from build123d import *

# Parameters (mm, degrees)
SKETCH1_R           = 31.0896
BOSS_EXTRUDE1_DEPTH = 16.002
BOSS_EXTRUDE2_START = -6.35
BOSS_EXTRUDE2_DEPTH = 6.35
FILLET2_R           = 6.35
CUT_EXTRUDE2_REACH  = 96.198
SKETCH4_R           = 1.778
SKETCH4_R_2         = 6.35
SKETCH7_R           = 2.0193
CUT_EXTRUDE4_DEPTH  = 95.197625109
FILLET7_R           = 6.35
FILLET8_R           = 41.148
CUT_EXTRUDE5_DEPTH  = 12.7
FILLET9_R           = 2.54
SKETCH9_R           = 6.35
CUT_EXTRUDE6_DEPTH  = 3.302
FILLET10_R          = 3.556


# Some blends are built 0.0001 mm under size
with BuildPart() as part:
    # Sketch1 → Boss-Extrude1 (new body)
    with BuildSketch(Plane(origin=(0, 0, 0), x_dir=(1, 0, 0), z_dir=(0, 1, 0))):
        with Locations(Location((0, 0, 0), (0, 0, 270))):
            Circle(SKETCH1_R)
    extrude(amount=BOSS_EXTRUDE1_DEPTH)

    # Sketch2 → Boss-Extrude2 (add)
    with BuildSketch(Plane(origin=(0, 16.002, 0), x_dir=(1, 0, 0), z_dir=(0, 1, 0)).offset(BOSS_EXTRUDE2_START)):
        with BuildLine():
            Line((-31.0896, 0), (-31.0896, 41.148))
            Line((-31.0896, 41.148), (83.2104, 41.148))
            Line((83.2104, 41.148), (83.2104, 15.748))
            Line((83.2104, 15.748), (31.0896, 15.748))
            Line((31.0896, 15.748), (31.0896, 0))
            ThreePointArc((31.0896, 0), (0, -31.0896), (-31.0896, 0))
        make_face()
    extrude(amount=BOSS_EXTRUDE2_DEPTH)

    # Fillet2
    fillet2_edges = [part.edges().sort_by_distance(p)[0] for p in [
        (31.0896, 12.827, -15.748),
    ]]
    fillet(fillet2_edges, radius=FILLET2_R)

    # Sketch4 → Cut-Extrude2 (cut, up to next)
    with BuildSketch(Plane(origin=(0, 16.002, 0), x_dir=(1, 0, 0), z_dir=(0, 1, 0)), mode=Mode.PRIVATE) as cut_extrude2_sk1:
        with Locations(Location((61.411202787, 35.362797213, 0), (0, 0, 270))):
            Circle(SKETCH4_R)
    cut_extrude2_tool1 = extrude(cut_extrude2_sk1.sketch, amount=-CUT_EXTRUDE2_REACH, mode=Mode.PRIVATE) & part.part
    # Sketch4 → Cut-Extrude2 (cut, up to next)
    with BuildSketch(Plane(origin=(0, 16.002, 0), x_dir=(1, 0, 0), z_dir=(0, 1, 0)), mode=Mode.PRIVATE) as cut_extrude2_sk2:
        with Locations(Location((75.240797213, 35.362797213, 0), (0, 0, 270))):
            Circle(SKETCH4_R)
    cut_extrude2_tool2 = extrude(cut_extrude2_sk2.sketch, amount=-CUT_EXTRUDE2_REACH, mode=Mode.PRIVATE) & part.part
    # Sketch4 → Cut-Extrude2 (cut, up to next)
    with BuildSketch(Plane(origin=(0, 16.002, 0), x_dir=(1, 0, 0), z_dir=(0, 1, 0)), mode=Mode.PRIVATE) as cut_extrude2_sk3:
        with Locations(Location((75.240797213, 21.533202787, 0), (0, 0, 270))):
            Circle(SKETCH4_R)
    cut_extrude2_tool3 = extrude(cut_extrude2_sk3.sketch, amount=-CUT_EXTRUDE2_REACH, mode=Mode.PRIVATE) & part.part
    # Sketch4 → Cut-Extrude2 (cut, up to next)
    with BuildSketch(Plane(origin=(0, 16.002, 0), x_dir=(1, 0, 0), z_dir=(0, 1, 0)), mode=Mode.PRIVATE) as cut_extrude2_sk4:
        with Locations(Location((68.326, 28.448, 0), (0, 0, 270))):
            Circle(SKETCH4_R_2)
    cut_extrude2_tool4 = extrude(cut_extrude2_sk4.sketch, amount=-CUT_EXTRUDE2_REACH, mode=Mode.PRIVATE) & part.part
    # Sketch4 → Cut-Extrude2 (cut, up to next)
    with BuildSketch(Plane(origin=(0, 16.002, 0), x_dir=(1, 0, 0), z_dir=(0, 1, 0)), mode=Mode.PRIVATE) as cut_extrude2_sk5:
        with Locations(Location((61.411202787, 21.533202787, 0), (0, 0, 270))):
            Circle(SKETCH4_R)
    cut_extrude2_tool5 = extrude(cut_extrude2_sk5.sketch, amount=-CUT_EXTRUDE2_REACH, mode=Mode.PRIVATE) & part.part
    add(cut_extrude2_tool1.solids().sort_by_distance((61.411203, 16.002, -35.362797))[0], mode=Mode.SUBTRACT)
    add(cut_extrude2_tool2.solids().sort_by_distance((75.240797, 16.002, -35.362797))[0], mode=Mode.SUBTRACT)
    add(cut_extrude2_tool3.solids().sort_by_distance((75.240797, 16.002, -21.533203))[0], mode=Mode.SUBTRACT)
    add(cut_extrude2_tool4.solids().sort_by_distance((68.326, 16.002, -28.448))[0], mode=Mode.SUBTRACT)
    add(cut_extrude2_tool5.solids().sort_by_distance((61.411203, 16.002, -21.533203))[0], mode=Mode.SUBTRACT)

    # Sketch7 → Cut-Extrude4 (cut, through all)
    with BuildSketch(Plane(origin=(0, 0, 0), x_dir=(1, 0, 0), z_dir=(0, 1, 0))):
        with BuildLine():
            ThreePointArc((27.94, 0), (22.235278576, 16.918510179), (7.450666667, 26.928259621))
            Line((7.450666667, 26.928259621), (4.402666667, 15.912153412))
            ThreePointArc((4.402666667, 15.912153412), (13.139028249, 9.997301469), (16.51, 0))
            ThreePointArc((16.51, 0), (13.139028249, -9.997301469), (4.402666667, -15.912153412))
            Line((4.402666667, -15.912153412), (7.450666667, -26.928259621))
            ThreePointArc((7.450666667, -26.928259621), (22.235278576, -16.918510179), (27.94, 0))
        make_face()
        with BuildLine():
            Line((-15.912153412, -4.402666667), (-26.928259621, -7.450666667))
            ThreePointArc((-26.928259621, -7.450666667), (-19.756563466, -19.756563466), (-7.450666667, -26.928259621))
            Line((-7.450666667, -26.928259621), (-4.402666667, -15.912153412))
            ThreePointArc((-4.402666667, -15.912153412), (-11.674332957, -11.674332957), (-15.912153412, -4.402666667))
        make_face()
        with BuildLine():
            Line((-4.402666667, 15.912153412), (-7.450666667, 26.928259621))
            ThreePointArc((-7.450666667, 26.928259621), (-19.756563466, 19.756563466), (-26.928259621, 7.450666667))
            Line((-26.928259621, 7.450666667), (-15.912153412, 4.402666667))
            ThreePointArc((-15.912153412, 4.402666667), (-11.674332957, 11.674332957), (-4.402666667, 15.912153412))
        make_face()
        with Locations(Location((-19.05, 0, 0), (0, 0, 270))):
            Circle(SKETCH7_R)
        with Locations(Location((0, -19.05, 0), (0, 0, 270))):
            Circle(SKETCH7_R)
        with Locations(Location((0, 19.05, 0), (0, 0, 270))):
            Circle(SKETCH7_R)
    extrude(amount=CUT_EXTRUDE4_DEPTH, mode=Mode.SUBTRACT)

    # Fillet7
    # the kernel refuses this fillet: 6.35 mm, written as the material it adds along each edge
    with BuildSketch(Plane(origin=(-26.928259621, 0, -7.450666667), x_dir=(0.40702884348062, 0, -0.9134153056385845), z_dir=(0, 1, 0)), Plane(origin=(-7.450666667, 0, 26.928259621), x_dir=(-0.9134153056385848, 0, -0.40702884348061963), z_dir=(0, 1, 0))) as fillet7_piece_1:
        with BuildLine():
            CenterArc((7.365726845, -6.279391075), FILLET7_R, 81.447682412, 107.104635177)
            Line((1.086335771, -7.223715029), (0, 0))
            ThreePointArc((0, 0), (4.1550254, 0.310679271), (8.3100508, 0))
        make_face()
    extrude(amount=16.002)
    with BuildSketch(Plane(origin=(-7.450666667, 0, -26.928259621), x_dir=(0.26666666666666705, 0, 0.9637888196533972), z_dir=(0, 1, 0)), Plane(origin=(7.450666667, 0, 26.928259621), x_dir=(-0.26666666666666733, 0, -0.9637888196533971), z_dir=(0, 1, 0)), Plane(origin=(-26.928259621, 0, 7.450666667), x_dir=(0.9637888196533975, 0, -0.26666666666666644), z_dir=(0, 1, 0))) as fillet7_piece_2:
        with BuildLine():
            CenterArc((7.304942452, -6.35), FILLET7_R, 90, 107.104635177)
            ThreePointArc((1.235807879, -8.217647059), (0.310679271, -4.1550254), (0, 0))
            Line((0, 0), (7.304942452, 0))
        make_face()
    extrude(amount=16.002)
    with BuildSketch(Plane(origin=(-4.402666667, 0, -15.912153412), x_dir=(-0.916852417954672, 0, 0.39922630636103035), z_dir=(0, 1, 0)), Plane(origin=(4.402666667, 0, 15.912153412), x_dir=(0.9168524179546733, 0, -0.39922630636102746), z_dir=(0, 1, 0)), Plane(origin=(-15.912153412, 0, 4.402666667), x_dir=(0.39922630636102946, 0, 0.9168524179546725), z_dir=(0, 1, 0))) as fillet7_piece_3:
        with BuildLine():
            CenterArc((5.522661099, -6.287214109), FILLET7_R, 98.063810107, 73.872379787)
            Line((-0.76455301, -5.396462319), (0, 0))
            ThreePointArc((0, 0), (2.315954654, -0.163243317), (4.631909309, 0))
        make_face()
    extrude(amount=16.002)
    with BuildSketch(Plane(origin=(4.402666667, 0, -15.912153412), x_dir=(0.26666666666666416, 0, -0.9637888196533979), z_dir=(0, 1, 0))) as fillet7_piece_4:
        with BuildLine():
            CenterArc((5.450352912, -6.35), FILLET7_R, 90, 73.872379787)
            ThreePointArc((-0.649745119, -4.586111111), (-0.163243317, -2.315954654), (0, 0))
            Line((0, 0), (5.450352912, 0))
        make_face()
    extrude(amount=16.002)
    with BuildSketch(Plane(origin=(7.450666667, 0, -26.928259621), x_dir=(-0.2666666666666666, 0, 0.9637888196533974), z_dir=(0, 1, 0))) as fillet7_piece_5:
        with BuildLine():
            CenterArc((7.304942452, 6.35), FILLET7_R, 162.895364823, 107.104635177)
            ThreePointArc((1.235807879, 8.217647059), (0.310679271, 4.1550254), (0, 0))
            Line((0, 0), (7.304942452, 0))
        make_face()
    extrude(amount=16.002)
    with BuildSketch(Plane(origin=(-4.402666667, 0, 15.912153412), x_dir=(-0.9168524179546729, 0, -0.3992263063610288), z_dir=(0, 1, 0)), Plane(origin=(-15.912153412, 0, -4.402666667), x_dir=(0.39922630636102996, 0, -0.9168524179546723), z_dir=(0, 1, 0))) as fillet7_piece_6:
        with BuildLine():
            CenterArc((5.522661099, 6.287214109), FILLET7_R, 188.063810107, 73.872379787)
            Line((-0.76455301, 5.396462319), (0, 0))
            ThreePointArc((0, 0), (2.315954654, 0.163243317), (4.631909309, 0))
        make_face()
    extrude(amount=16.002)

    # Fillet8
    fillet8_edges = [part.edges().sort_by_distance(p)[0] for p in [
        (-31.0896, 12.827, -41.148),
    ]]
    fillet(fillet8_edges, radius=FILLET8_R - 0.0001)  # a hair under: the kernel refuses the full size

    # Sketch8 → Cut-Extrude5 (cut)
    with BuildSketch(Plane.XZ):
        with BuildLine():
            Line((-10.414, 10.414), (10.414, 10.414))
            ThreePointArc((10.414, 10.414), (20.828, 0), (10.414, -10.414))
            Line((10.414, -10.414), (-10.414, -10.414))
            Line((-10.414, -10.414), (-10.414, 10.414))
        make_face()
    extrude(amount=-CUT_EXTRUDE5_DEPTH, mode=Mode.SUBTRACT)

    # Fillet9
    # the kernel refuses this fillet: 2.54 mm, written as the material it takes off along each edge
    with BuildSketch(Plane(origin=(13.087195122, 12.7, 10.065059555), x_dir=(-0.7525451578932851, 0, 0.658540648199768), z_dir=(0, -1, 0))) as fillet9_piece_1:
        with BuildLine():
            CenterArc((7.288242174, 2.538935053), FILLET9_R, 131.188669075, 137.152126286)
            Line((5.615548928, 4.450399754), (5.448279603, 4.641546224))
            ThreePointArc((5.448279603, 4.641546224), (2.074222188, 1.688960676), (-0.1125988, 0.227678524))
            Line((-0.1125988, 0.227678524), (-0.049545453, -0.249120951))
            ThreePointArc((-0.049545453, -0.249120951), (6.014734512, -0.336617786), (7.207343199, -0.253893505))
            Line((7.207343199, -0.253893505), (7.214697651, 0))
        make_face()
    extrude(amount=30.736744128, mode=Mode.SUBTRACT)
    with BuildSketch(Plane(origin=(13.087195122, 12.7, -10.065059555), x_dir=(-0.7525451578933744, 0, -0.658540648199666), z_dir=(0, -1, 0))) as fillet9_piece_2:
        with BuildLine():
            CenterArc((7.288242174, -2.538935053), FILLET9_R, 91.659204639, 137.152126286)
            Line((5.615548928, -4.450399754), (5.448279603, -4.641546224))
            ThreePointArc((5.448279603, -4.641546224), (2.074222188, -1.688960676), (-0.1125988, -0.227678524))
            Line((-0.1125988, -0.227678524), (-0.049545453, 0.249120951))
            ThreePointArc((-0.049545453, 0.249120951), (6.014734512, 0.336617786), (7.207343199, 0.253893505))
            Line((7.207343199, 0.253893505), (7.214697651, 0))
        make_face()
    extrude(amount=30.736744128, mode=Mode.SUBTRACT)

    # Sketch9 → Cut-Extrude6 (cut)
    with BuildSketch(Plane.XZ.offset(-12.7)):
        with Locations(Location((0, 0, 0), (0, 0, 270))):
            Circle(SKETCH9_R)
    extrude(amount=-CUT_EXTRUDE6_DEPTH, mode=Mode.SUBTRACT)

    # Fillet10
    fillet10_edges = [part.edges().sort_by_distance(p)[0] for p in [
        (-10.414, 6.35, -10.414),
        (-10.414, 6.35, 10.414),
    ]]
    fillet(fillet10_edges, radius=FILLET10_R)


solid = part.part
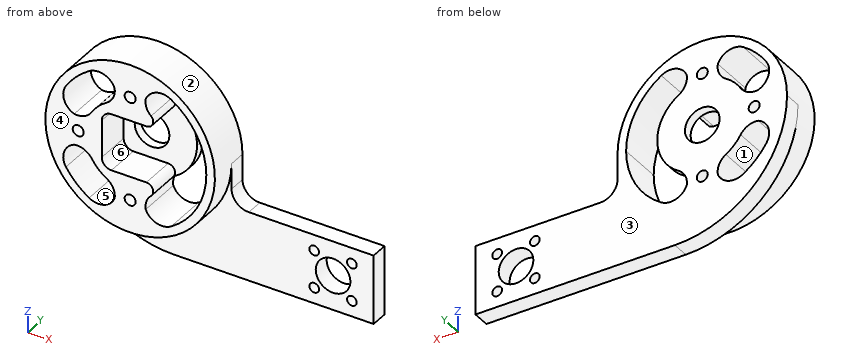
The listing builds one solid part. Answer for the finished solid, in the listing's coordinates (mm). Face numbers are marked on the shaded views. A direction names the side the tool comes from. Coordinates: 2 decimals unless noted, no trailing zeros. Loops run counter-clockwise (first coordinate to the right, second up) from the corner with the lowest first, then second, coordinate; pieces in that order, holes last. Notation, with made-up numbers: (85.25, 38.25) -> (123.25, 38.25) arc R30 ccw to (123.25, 69.25) -> close; hole circle Ø8 at (52, 31.25). An arc over 180 degrees is marked (long way). Write item = value, one per line. Start each with the question number.
1) A cutting plane is placed at C-C (x = -19.05). Give the vertices of the cut face in (y, z), then the cut area to 3 significant figures.
2) A cutting plane is placed at B-B (x = 12). Give the vertices of the cut face in (y, z).
3) The mould has two halves that part along X. Classify the marked faces 1, 2 and 3: released by +X, released by -X, zero draft, split by the parting line, or undercut.
4) Given pin 1 Ø4 at (y, z) = (7, -19.5) entering from +X; pin 2 Ø1.5 at (y, z) = (9.5, -3) entering from +X; pin 3 Ø5.5 at (x, z) = (75.24, -21.53) entering from +Y; pin 4 Ø4 at (x, z) = (61.41, -35.36) entering from -Y, each flat-ended and moving along its own axis, determine where each tip first touches the part or whether it passes through.
5) A cutting plane is placed at A-A (z = 19.05). Give the vertices of the cut face in (x, y), then the cut area to 3 significant figures.
6) Straight lines are drawn through the part: line 1 (Z direction, x = 0, y = 8); line 2 (X direction, y = 10.5, z = 14); line 3 (Z direction, x = -9.5, y = 8.5). For each, find the intervals that lie inside material, in ascending order. Write a range as from..to.
7) A cutting plane is placed at D-D (z = -3.5). Give the vertices of the cut face in (x, y).
8) A tool of negligible diameter and unlimited length cuts with its end or side. For the marked faces 4, 5 and 6, from which of +Z, -Z, +X, -X, +Y, -Y can it reach the whole face along a straight path? Write none if from no direction.
Responses:
q1.outline = (0, -24.57) -> (9.65, -24.57) -> (9.65, -29.08) -> (16, -29.08) -> (16, -20.44) -> (0, -20.44) -> close; (0, -5.64) -> (16, -5.64) -> (16, -2.02) -> (0, -2.02) -> close; (0, 2.02) -> (16, 2.02) -> (16, 5.64) -> (0, 5.64) -> close; (0, 20.44) -> (16, 20.44) -> (16, 24.57) -> (0, 24.57) -> close
q1.area = 277 mm²
q2.outline = (0, -28.68) -> (9.65, -28.68) -> (9.65, -41.15) -> (16, -41.15) -> (16, -24.53) -> (0, -24.53) -> close; (0, 24.53) -> (16, 24.53) -> (16, 28.68) -> (0, 28.68) -> close; (12.7, -11.34) -> (16, -11.34) -> (16, 11.34) -> (12.7, 11.34) -> close
q3.face_1 = undercut
q3.face_2 = split by the parting line
q3.face_3 = zero draft
q4.pin_1 = 25.7
q4.pin_2 = 31.09
q4.pin_3 = 16
q4.pin_4 = 9.65
q5.outline = (-24.57, 0) -> (-20.44, 0) -> (-20.44, 16) -> (-24.57, 16) -> close; (-5.64, 0) -> (-2.02, 0) -> (-2.02, 16) -> (-5.64, 16) -> close; (2.02, 0) -> (5.64, 0) -> (5.64, 16) -> (2.02, 16) -> close; (20.44, 0) -> (24.57, 0) -> (24.57, 16) -> (20.44, 16) -> close
q5.area = 248 mm²
q6.line_1 = -31.09..-21.07, -17.03..-10.41, 10.41..17.03, 21.07..31.09
q6.line_2 = -27.76..-24.08, -8.75..8.25, 24.18..27.76
q6.line_3 = -29.6..-24.18, -13.5..-9.24, 9.24..13.5, 24.18..29.6
q7.outline = (-30.94, 9.65) -> (-30.89, 9.65) -> (-30.89, 0) -> (-10.41, 0) -> (-10.41, 12.7) -> (-5.3, 12.7) -> (-5.3, 16) -> (-30.94, 16) -> close; (5.3, 12.7) -> (16.13, 12.7) -> (16.13, 16) -> (5.3, 16) -> close; (27.72, 0) -> (30.89, 0) -> (30.89, 9.65) -> (31.09, 9.65) -> (31.09, 16) -> (27.72, 16) -> close
q8.face_4 = +Z, -Z, +X, -X, -Y
q8.face_5 = +Y, -Y
q8.face_6 = -Y
